Design review of the part built by this model. Coordinates are the model's own, in mm. A direction names the side the tool comes from. Coordinates: 2 decimals unless noted, no trailing zeros. Write each loop counter-clockwise with the first axis right and the second up, starting at its lowest first coordinate (ties: lowest second). Pieces come first, ordered by that corner, then holes.
Q1. Add section B-B, the plane y = 6.25. Give the number of separate pieces and of enclosed holes in the cut face, plus the area to 3 significant figures.
Q2. The part is to be moulded in two halves that separate along Z. For faces 4 (the face through (0, 0, 0)), 5 (the face through (0, 3, -2.875)), 6 (the face through (0, 5, 2.125)), 7 (the face through (0, 4, -2.075)), say which applies: +Z half, -Z half, draft (parallel to the pull), parting line (faces both ways), or undercut.
Q3. To check wall thickness, follow probe 1 along X at (y, z) = (1.5, 0.6); probe 2 along Z at (x, y) = (1, 5) (3 decimals); probe 3 along Z at (x, y) = (-0.25, 1) (3 decimals). State the ranges of each line that lie inside material, in increasing order.
Q4. Add section C-C, the plane x = -4.5. Give the boundary of the cut face in (y, z) (3 decimals), plus the area to 4 significant figures.
Q5. Add section D-D, the plane y = -0.5. Give the boundary of the cut face in (x, z) (3 decimals), plus the area to 3 significant figures.
Q6. Add section A-A, the plane y = 2.5. Give the boundary of the cut face in (x, z) (3 decimals).
Q7. Machinability: for faces 1 (the face through (4.15, 4, 0)), 2 (the face through (4.95, 3, 0)), 3 (the face through (-4, 5, 2.125)), which of the approach directions +Z, -Z, +X, -X, +Y, -Y give a long, thin tool a straight path to every point of the face, cutting with its end or side? Answer none if there is none.
Q8. Clearance check with flat-ended pins moving along their axes: pin 1 Ø0.5 at (y, z) = (-2, 0.5) entering from -X; pin 2 Ø3 at (x, z) = (-2.5, 0.5) entering from +Y; pin 3 Ø1 at (y, z) = (-1.5, 0) entering from +X. State where each tip first meets the part, or that it passes through.
from build123d import *

# Parameters (mm, degrees)
SKETCH1_W                = 9.9
SKETCH1_H                = 5.75
BOSS_EXTRUDE1_DEPTH      = 7
SHELL1_T                 = -0.8
SKETCH2_W                = 1.25
SKETCH2_H                = 3.2
CUT_EXTRUDE1_DEPTH       = 10.9
CUT_EXTRUDE2_REACH       = 7.75
SKETCH3_W                = 1.7
SKETCH3_H                = 3.8
SKETCH4_W                = 0.64
SKETCH4_H                = 0.64
BOSS_EXTRUDE2_DEPTH      = 3.45
BOSS_EXTRUDE2_DEPTH_BACK = 6.75
CHAMFER1_SIZE            = 0.2


with BuildPart() as part:
    # Sketch1 → Boss-Extrude1 (new body)
    with BuildSketch(Plane(origin=(0, 0, 0), x_dir=(1, 0, 0), z_dir=(0, 1, 0))):
        Rectangle(SKETCH1_W, SKETCH1_H)
    extrude(amount=BOSS_EXTRUDE1_DEPTH)

    # Shell1
    shell1_openings = [part.faces().sort_by_distance(p)[0] for p in [
        (0, 7, 0),
    ]]
    offset(amount=SHELL1_T, openings=shell1_openings, kind=Kind.INTERSECTION)

    # Sketch2 → Cut-Extrude1 (cut, through all)
    with BuildSketch(Plane(origin=(4.95, 0, 0), x_dir=(0, 0, -1), z_dir=(1, 0, 0))):
        with Locations((-1.5, 5.4)):
            Rectangle(SKETCH2_W, SKETCH2_H)
    extrude(amount=-CUT_EXTRUDE1_DEPTH, mode=Mode.SUBTRACT)

    # Sketch3 → Cut-Extrude2 (cut, up to next)
    with BuildSketch(Plane.XY.offset(2.875), mode=Mode.PRIVATE) as cut_extrude2_sk1:
        with Locations((-2.2, 5.1)):
            Rectangle(SKETCH3_W, SKETCH3_H)
    cut_extrude2_tool1 = extrude(cut_extrude2_sk1.sketch, amount=-CUT_EXTRUDE2_REACH, mode=Mode.PRIVATE) & part.part
    add(cut_extrude2_tool1.solids().sort_by_distance((-2.2, 5.1, 2.875))[0], mode=Mode.SUBTRACT)
    # Sketch3 → Cut-Extrude2 (cut, up to next)
    with BuildSketch(Plane.XY.offset(2.875), mode=Mode.PRIVATE) as cut_extrude2_sk2:
        with Locations((2.2, 5.1)):
            Rectangle(SKETCH3_W, SKETCH3_H)
    cut_extrude2_tool2 = extrude(cut_extrude2_sk2.sketch, amount=-CUT_EXTRUDE2_REACH, mode=Mode.PRIVATE) & part.part
    add(cut_extrude2_tool2.solids().sort_by_distance((2.2, 5.1, 2.875))[0], mode=Mode.SUBTRACT)

    # Sketch4 → Boss-Extrude2 (add, two sides)
    with BuildSketch(Plane.XZ) as boss_extrude2_sk:
        with Locations((-2.5, 0.525)):
            Rectangle(SKETCH4_W, SKETCH4_H)
        with Locations((0, 0.525)):
            Rectangle(SKETCH4_W, SKETCH4_H)
        with Locations((2.5, 0.525)):
            Rectangle(SKETCH4_W, SKETCH4_H)
    extrude(amount=BOSS_EXTRUDE2_DEPTH)
    extrude(boss_extrude2_sk.sketch, amount=-BOSS_EXTRUDE2_DEPTH_BACK)

    # Chamfer1
    chamfer1_edges = [part.edges().sort_by_distance(p)[0] for p in [
        (0.32, 6.75, 0.525),
        (0, 6.75, 0.205),
        (-0.32, 6.75, 0.525),
        (0, 6.75, 0.845),
        (0.32, -3.45, 0.525),
        (0, -3.45, 0.845),
        (-0.32, -3.45, 0.525),
        (0, -3.45, 0.205),
        (2.82, 6.75, 0.525),
        (2.5, 6.75, 0.205),
        (2.18, 6.75, 0.525),
        (2.5, 6.75, 0.845),
        (2.82, -3.45, 0.525),
        (2.5, -3.45, 0.845),
        (2.18, -3.45, 0.525),
        (2.5, -3.45, 0.205),
        (-2.18, 6.75, 0.525),
        (-2.5, 6.75, 0.205),
        (-2.82, 6.75, 0.525),
        (-2.5, 6.75, 0.845),
        (-2.18, -3.45, 0.525),
        (-2.5, -3.45, 0.845),
        (-2.82, -3.45, 0.525),
        (-2.5, -3.45, 0.205),
    ]]
    chamfer(chamfer1_edges, length=CHAMFER1_SIZE)


solid = part.part
Here are the results:
1. separate pieces: 7
1. enclosed holes: 0
1. area: 18.7 mm2
2. face 4: draft
2. face 5: -Z half
2. face 6: undercut
2. face 7: undercut
3. probe 1: x = -4.95 to -4.15, -2.82 to -2.18, -0.32 to 0.32, 2.18 to 2.82, 4.15 to 4.95
3. probe 2: z = -2.875 to -2.075, 2.125 to 2.875
3. probe 3: z = -2.875 to -2.075, 0.205 to 0.845, 2.075 to 2.875
4. outline: (0, -2.875) - (7, -2.875) - (7, 0.875) - (3.8, 0.875) - (3.8, 2.125) - (7, 2.125) - (7, 2.875) - (0, 2.875) - close
4. area: 36.25 mm2
5. outline: (-2.82, 0.205) - (-2.18, 0.205) - (-2.18, 0.845) - (-2.82, 0.845) - close; (-0.32, 0.205) - (0.32, 0.205) - (0.32, 0.845) - (-0.32, 0.845) - close; (2.18, 0.205) - (2.82, 0.205) - (2.82, 0.845) - (2.18, 0.845) - close
5. area: 1.23 mm2
6. outline: (-4.95, -2.875) - (4.95, -2.875) - (4.95, 2.875) - (-4.95, 2.875) - close; (-2.82, 0.205) - (-2.18, 0.205) - (-2.18, 0.845) - (-2.82, 0.845) - close; (-0.32, 0.205) - (0.32, 0.205) - (0.32, 0.845) - (-0.32, 0.845) - close; (2.18, 0.205) - (2.82, 0.205) - (2.82, 0.845) - (2.18, 0.845) - close; hole (-4.15, -2.075) - (4.15, -2.075) - (4.15, 2.075) - (-4.15, 2.075) - close
7. face 1: +Y
7. face 2: +Z, -Z, +X, +Y, -Y
7. face 3: +X, -X, +Y
8. pin 1: stops at x = -2.82
8. pin 2: stops at y = 6.75
8. pin 3: stops at x = 2.82
